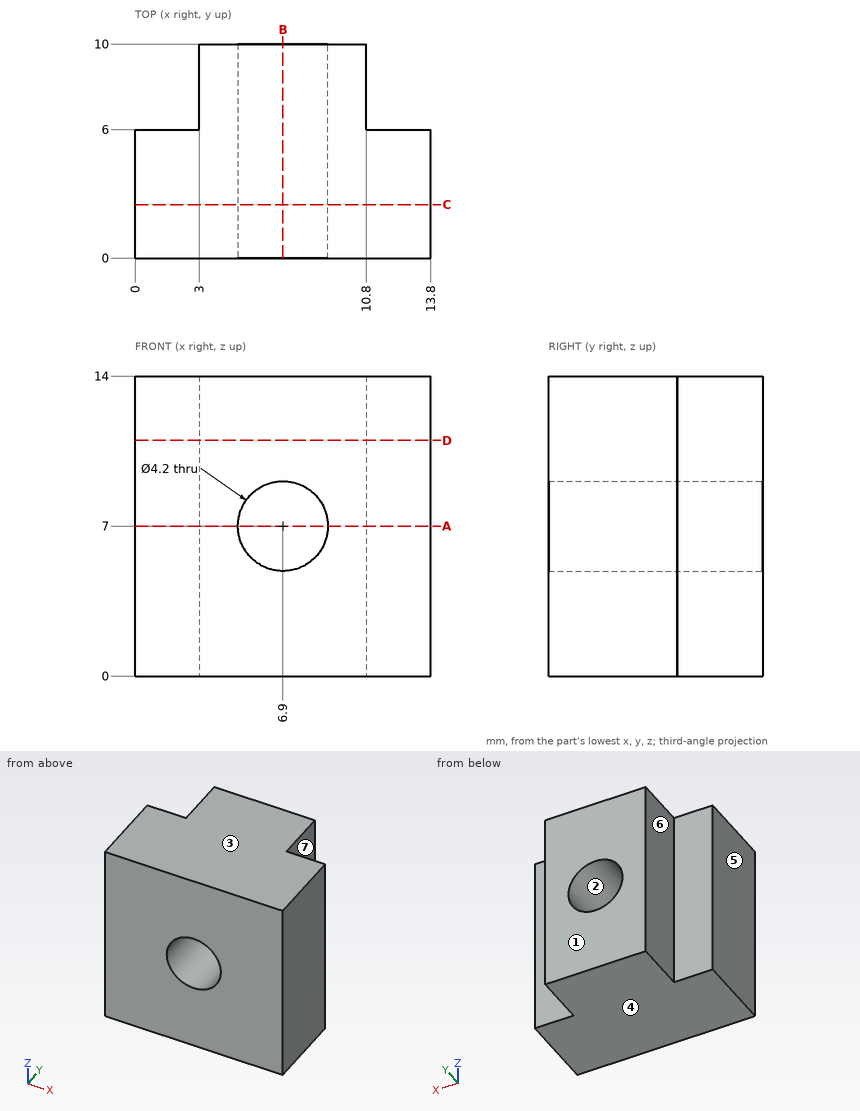
Could you check a few things on this drawing? It's one solid part, dimensions in mm from its lowest x, y, z. A direction names the side the tool comes from. Coordinates: 2 decimals unless noted, no trailing zeros. Order: outer loops, then holes, each group sorted by start corner. A loop starts at its lowest first (then second) coordinate and runs counter-clockwise, first axis right, second up. Notation, with made-up numbers: (22.5, 43.5) - (56.5, 43.5) arc R9 cw to (56.5, 54.5) - close; hole circle Ø3 at (28, 19.5). An arc over 180 degrees is marked (long way). Answer as a JSON object with one key per item and string values. Group by question number.
Q1. Imagine slicing it at C-C (y = 2.5). Please give me the cut outline in (x, z), and give its area (3 significant figures).
Q2. Imagine slicing it at B-B (x = 6.9). Please give me the cut outline in (y, z), and give its area (3 significant figures).
Q3. Imagine slicing it at D-D (z = 11). Please give me the cut outline in (x, y), and give its area (3 significant figures).
Q4. Will these pins go through, and if not, where does the flat tip stop? P1, Ø2.5, axis at x = 1, z = 4, coming from the +Y side; P2, Ø5, axis at x = 6.9, z = 7, coming from the -Y side; P3, Ø1.2, axis at y = 8.5, z = 7, coming from the -X side; P4, Ø4.5, axis at y = 8.5, z = 7.5, coming from the +X side.
Q5. Imagine slicing it at A-A (z = 7). Please give me the cut outline in (x, y), and give its area (3 significant figures).
Q6. On a 3-axis mill with a long thin cutter (end or side, diameter ignored), from which of +Z, -Z, +X, -X, +Y, -Y can I reach the whole of each face in a straight line? I mean the marked faces 5, 6 and 7. Say none if no direction works.
Q7. I need wall thicknesses on line 1 (Z direction, x = 6.9, y = 3); line 2 (X direction, y = 2, z = 8); line 3 (Y direction, x = 11, z = 12.5). Which ranges of each line are inside material? Lowest first, please. Write a range as from..to.
Q8. We'd pull the mould along Z, two halves only. Please class the marked faces 1, 2, 3 and 4: +Z half, -Z half, draft (parallel to the pull), parting line (faces both ways), or undercut.
Determined:
{
 "1": {"outline": "(0, 0) - (13.8, 0) - (13.8, 14) - (0, 14) - close; hole circle Ø4.2 at (6.9, 7)", "area": "179 mm2"},
 "2": {"outline": "(0, 0) - (10, 0) - (10, 4.9) - (0, 4.9) - close; (0, 9.1) - (10, 9.1) - (10, 14) - (0, 14) - close", "area": "98.0 mm2"},
 "3": {"outline": "(0, 0) - (13.8, 0) - (13.8, 6) - (10.8, 6) - (10.8, 10) - (3, 10) - (3, 6) - (0, 6) - close", "area": "114 mm2"},
 "4": {"P1": "stops at y = 6", "P2": "stops at y = 0", "P3": "stops at x = 3", "P4": "stops at x = 10.8"},
 "5": {"outline": "(0, 0) - (4.8, 0) - (4.8, 10) - (3, 10) - (3, 6) - (0, 6) - close; (9, 0) - (13.8, 0) - (13.8, 6) - (10.8, 6) - (10.8, 10) - (9, 10) - close", "area": "72.0 mm2"},
 "6": {"face 5": "+Z, -Z, -X, +Y, -Y", "face 6": "+Z, -Z, -X, +Y", "face 7": "+Z, -Z, +X, +Y"},
 "7": {"line 1": "z = 0..4.9, 9.1..14", "line 2": "x = 0..5.05, 8.75..13.8", "line 3": "y = 0..6"},
 "8": {"face 1": "draft", "face 2": "undercut", "face 3": "+Z half", "face 4": "-Z half"}
}
